Read the model definition and answer for the solid it produces. Units are mm, in the model's axes. Round coordinates to 2 decimals unless told otherwise and drop trailing zeros. Write each loop counter-clockwise with the first axis right and the second up, starting at its lowest first coordinate (ties: lowest second). Pieces come first, ordered by that corner, then holes. Notation, with made-up numbers: (-33.75, -27) - (-22.75, -27) arc R29 ccw to (-22.75, -4) - close; hole circle Ø6 at (21.25, -14.5). An arc over 180 degrees is marked (long way). One line per item, written item: value. Start each with the question number.
(1) A cutting plane is placed at A-A, the plane x = -9.75. Determine the outline of the cut face in (y, z), plus the area to 3 significant figures.
(2) A cutting plane is placed at B-B, the plane x = -4.75. Determine the outline of the cut face in (y, z).
(3) The mould has two halves that part along Z. Classify faces 1 (the face through (-6, 0, -6)), 2 (the face through (-11, 0, 0)), 3 (the face through (0, -6.1, 2)), 4 (the face through (-6.35, -7, -1.56)): +Z half, -Z half, draft (parallel to the pull), parting line (faces both ways), or undercut.
(4) Flat-ended cylindrical pins translate along their axes: pin 1 Ø1 at (y, z) = (-2, 2.5) entering from +X; pin 2 Ø5 at (y, z) = (0.5, 3) entering from -X; pin 3 Ø5 at (x, y) = (-5.5, 2) entering from -Z. Find the tip coordinate at first contact, or state that the pin passes through.
(5) Find the intervals of material crossed by L1, parallel to Y at x = -3.75, z = -2.5; L2, parallel to Y at x = -3.25, z = 0; L3, parallel to Z at x = -10.75, y = -2.25, in increasing order.
Autodesk Inventor part; units mm, degrees
ref_plane "YZ Plane" through (0, 0, 0) normal (1, 0, 0) x (0, 1, 0)
ref_plane "XZ Plane" through (0, 0, 0) normal (0, 1, 0) x (-1, 0, 0)
ref_plane "XY Plane" through (0, 0, 0) normal (0, 0, 1) x (1, 0, 0)
sketch "Sketch1" plane through (0, 0, 0) normal (0, 1, 0) x (-1, 0, 0)
  line L0 (0, 0) -> (13, 0) construction
  line L1 (0.25, 6) -> (11, 6)
  line L2 (11, 6) -> (11, 0)
  line L3 (0, 6.25) -> (0, 6.8529)
  line L4 (13, 0) -> (13, 7.25) construction
  line L5 (12.2775, 7.2417) -> (0.2471, 7.1029)
  arc A0 (13, 0) -> (12.5284, 7.023) centre (-46.9979, -0.5017) ccw
  arc A1 (0.2471, 7.1029) -> (0, 6.8529) centre (0.25, 6.8529) ccw
  arc A2 (0, 6.25) -> (0.25, 6) centre (0.25, 6.25) ccw
  arc A3 (12.5284, 7.023) -> (12.2775, 7.2417) centre (12.2804, 6.9917) ccw
  line L6 (13, 0) -> (11, 0)
  point P0 (0, 6)
  point P1 (0, 7.1)
  point P2 (12.5, 7.2442)
  dimension "d0" = 13
  dimension "d1" = 11
  dimension "d2" = 6
  dimension "d3" = 1.1
  dimension "d5" = 2
  dimension "d6" = 7.25
  dimension "d7" = 60
  dimension "d8" = 0.5
  dimension "d9" = 0.25
revolve "Revolution1" add sketch "Sketch1" angle 360 about axis through (0, 0, 0) along (-1, 0, 0)
properties part number "12mm_Endcap" material "Rubber"
Here are the results:
1. outline: circle Ø14.43 at (0, 0); hole circle Ø12 at (0, 0)
1. area: 50.3 mm²
2. outline: circle Ø14.31 at (0, 0); hole circle Ø12 at (0, 0)
3. face 1: undercut
3. face 2: undercut
3. face 3: draft
3. face 4: parting line
4. pin 1: x = -11
4. pin 2: x = -12.99
4. pin 3: z = -7.18
5. L1: -6.69 to -5.45, 5.45 to 6.69
5. L2: -7.14 to -6, 6 to 7.14
5. L3: -6.86 to -5.56, 5.56 to 6.86
